Input: part model. Units: mm. Frame: model coordinates. Coordinates: 2 decimals unless noted, no trailing zeros. Loops run counter-clockwise (first coordinate to the right, second up) from the corner with the lowest first, then second, coordinate; pieces in that order, holes last. Notation, with made-up numbers: (49, -1) - (105, -1) arc R10 cw to (105, 11) - close; hole circle Ø9 at (29.25, -22). An arc over 180 degrees is marked (long way). Write item = value, one per line. Start each with the question number.
from build123d import *

# Parameters (mm, degrees)
F0_R     = 27
F0_R_2   = 19.25
F1_DEPTH = 8
F2_R     = 5
F3_R     = 0.5
F4_R     = 0.5


with BuildPart() as f1:
    # F0 (on Top) → F1 (new body)
    with BuildSketch(Plane.XY):
        Circle(F0_R)
        Circle(F0_R_2, mode=Mode.SUBTRACT)
    extrude(amount=F1_DEPTH)

    # F2
    f2_edges = [f1.edges().sort_by_distance(p)[0] for p in [
        (-27, 0, 8),
    ]]
    fillet(f2_edges, radius=F2_R)

    # F3
    f3_edges = [f1.edges().sort_by_distance(p)[0] for p in [
        (-19.25, 0, 8),
        (-19.25, 0, 0),
    ]]
    fillet(f3_edges, radius=F3_R)

    # F4
    f4_edges = [f1.edges().sort_by_distance(p)[0] for p in [
        (-27, 0, 0),
    ]]
    fillet(f4_edges, radius=F4_R)


solid = f1.part
Item 1: Cut plane A-A on x = 0. Return loops of the section in (y, z), plus the area to 3 significant figures.
Item 2: Cut plane C-C on z = 4.75. Return loops of the section in (x, y), plus the area to 3 significant figures.
Item 3: Ray query, line 1 (Y direction, x = 0, z = 2.25); line 2 (Y direction, x = -13, z = 7); line 3 (Z direction, x = -7.5, y = -21). Return the intervals inside material, ascending.
Item 4: Pull-direction query (Y, two-part tool) for faces 1 (the flat face through (-16, 12, 8)), 2 (the cylindrical face through (-5.85, -26.36, 1.73)), 3 (the cylindrical face through (-15.28, -11.71, 3.95)); classes: pulls with the +Y half, pulls with the -Y half, needs draft (parallel to the pull), parting line crosses it, or undercut.
Item 5: Pin query (flat end, axial travel): pin 1 (4 mm diameter, centred on y = -10.5, z = 4.5, fed in from -X); pin 2 (2 mm diameter, centred on x = -18, z = 3.5, fed in from -Y); pin 3 (1 mm diameter, centred on y = 0, z = 7, fed in from +X). Return the tip coordinate at first contact, or that it passes through.
Recorded:
q1.outline = (-27, 0.5) arc R0.5 ccw to (-26.5, 0) - (-19.75, 0) arc R0.5 ccw to (-19.25, 0.5) - (-19.25, 7.5) arc R0.5 ccw to (-19.75, 8) - (-22, 8) arc R5 ccw to (-27, 3) - close; (19.25, 0.5) arc R0.5 ccw to (19.75, 0) - (26.5, 0) arc R0.5 ccw to (27, 0.5) - (27, 3) arc R5 ccw to (22, 8) - (19.75, 8) arc R0.5 ccw to (19.25, 7.5) - close
q1.area = 113 mm²
q2.outline = circle Ø53.37 at (0, 0); hole circle Ø38.5 at (0, 0)
q2.area = 1,070 mm²
q3.line_1 = -27 to -19.25, 19.25 to 27
q3.line_2 = -21.35 to -14.2, 14.2 to 21.35
q3.line_3 = 0 to 7.99
q4.face_1 = needs draft
q4.face_2 = parting line crosses it
q4.face_3 = undercut
q5.pin_1 = -25.52
q5.pin_2 = -20.95
q5.pin_3 = 25.57
